Geometry check sheet. Reference: the model listing, model coordinates, mm. Round coordinates to 2 decimals unless told otherwise and drop trailing zeros. Order: outer loops, then holes, each group sorted by start corner. A loop starts at its lowest first (then second) coordinate and runs counter-clockwise, first axis right, second up.
(1) Gauge pin test, flat end, axial feed: P1, Ø2, axis at y = 1.5, z = 118.5, coming from the -X side. Record the tip position at first contact, or that the pin passes through.
(2) Cross-section at B-B on x = -1.25. Enter the section's corners in (y, z), and give its area (3 significant figures).
(3) Thickness scan on L1, parallel to X at y = -0.5, z = 294.5; L2, parallel to X at y = 1, z = 214. Record the ranges inside material, lowest first.
(4) Cross-section at A-A on z = 246.5. Enter the section's corners in (x, y).
(5) Cross-section at C-C on y = -2.25. Enter the section's corners in (x, z).
from build123d import *

# Parameters (mm, degrees)
SKETCH1_R           = 4
BOSS_EXTRUDE1_DEPTH = 287.5
SKETCH2_R           = 4
BOSS_EXTRUDE2_DEPTH = 45
SKETCH3_R           = 4
CUT_EXTRUDE1_DEPTH  = 65
SKETCH4_R           = 4
BOSS_EXTRUDE5_DEPTH = 13


with BuildPart() as part:
    # Sketch1 → Boss-Extrude1 (new body)
    with BuildSketch(Plane.XY):
        Circle(SKETCH1_R)
    extrude(amount=BOSS_EXTRUDE1_DEPTH)

    # Sketch2 → Boss-Extrude2 (add)
    with BuildSketch(Plane.XY.offset(287.5)):
        Circle(SKETCH2_R)
    extrude(amount=BOSS_EXTRUDE2_DEPTH)

    # Sketch3 → Cut-Extrude1 (cut)
    with BuildSketch(Plane(origin=(0, 0, 0), x_dir=(-1, 0, 0), z_dir=(0, 0, -1))):
        Circle(SKETCH3_R)
    extrude(amount=-CUT_EXTRUDE1_DEPTH, mode=Mode.SUBTRACT)

    # Sketch4 → Boss-Extrude5 (add)
    with BuildSketch(Plane(origin=(0, 0, 65), x_dir=(-1, 0, 0), z_dir=(0, 0, -1))):
        Circle(SKETCH4_R)
    extrude(amount=BOSS_EXTRUDE5_DEPTH)


solid = part.part
Found:
1. P1: stops at x = -3.97
2. outline: (-3.8, 52) - (3.8, 52) - (3.8, 332.5) - (-3.8, 332.5) - close
2. area: 2,130 mm2
3. L1: x = -3.97 to 3.97
3. L2: x = -3.87 to 3.87
4. outline: circle Ø8 at (0, 0)
5. outline: (-3.31, 52) - (3.31, 52) - (3.31, 332.5) - (-3.31, 332.5) - close
